For this review, take the finished solid that the model builds, in its own axes (mm). Round coordinates to 2 decimals unless told otherwise and drop trailing zeros. Write each loop counter-clockwise with the first axis right and the second up, starting at its lowest first coordinate (ties: lowest second). Pieces come first, ordered by that corner, then holes. Notation, with made-up numbers: (-33, -11.5) -> (0, -11.5) arc R19 ccw to (0, 25.5) -> close; hole circle Ø5 at (40.5, -15.5). An arc over 180 degrees is marked (long way). Answer in a Markdown table with one row per item. Add a question column.
Autodesk Inventor part; units mm, degrees
ref_plane "YZ Plane" through (0, 0, 0) normal (1, 0, 0) x (0, 1, 0)
ref_plane "XZ Plane" through (0, 0, 0) normal (0, 1, 0) x (-1, 0, 0)
ref_plane "XY Plane" through (0, 0, 0) normal (0, 0, 1) x (1, 0, 0)
sketch "Sketch1" plane through (0, 0, 0) normal (0, 0, 1) x (1, 0, 0)
  circle A0 centre (65.1069, 65.1069) radius 38.1 construction
  circle A1 centre (-56.1266, -56.1266) radius 25.4 construction
  circle A2 centre (0, 0) radius 53.975 construction
  line L0 (-38.1661, -38.1661) -> (38.1661, 38.1661) construction
  line L1 (65.1069, 65.1069) -> (-56.1266, -56.1266) construction
  line L2 (-4.3707, 6.2419) -> (-4.3707, 53.7978) construction
  line L3 (-213.7812, -81.5266) -> (651.6109, -81.5266) construction
  circle A3 centre (160.9392, -24.3766) radius 57.15 construction
  circle A4 centre (65.1069, 65.1069) radius 14.2875
  circle A5 centre (-56.1266, -56.1266) radius 14.2875
  circle A6 centre (-4.3707, 6.2419) radius 57.15 construction
  circle A7 centre (-56.1266, -56.1266) radius 20.6375 construction
  circle A8 centre (65.1069, 65.1069) radius 23.8125 construction
  circle A9 centre (-73.6972, 80.6773) radius 14.2875
  line L4 (-73.6972, 80.6773) -> (65.1069, 65.1069) construction
  circle A10 centre (65.1069, 65.1069) radius 14.3256 construction
  circle A11 centre (-56.1266, -56.1266) radius 14.3256 construction
  circle A12 centre (-109.5316, 9.8231) radius 14.2875
  line L5 (-56.1266, -56.1266) -> (-109.5316, 9.8231) construction
  circle A13 centre (-109.5316, 9.8231) radius 39.7002 construction
  circle A14 centre (-73.6972, 80.6773) radius 39.7002 construction
  line L6 (17.4877, 59.0466) -> (55.9992, 43.1049)
  line L7 (-39.0193, -44.5834) -> (-51.7448, -25.7239)
  arc A15 (17.4877, 59.0466) -> (-51.7448, -25.7239) centre (-4.3707, 6.2419) ccw
  line L8 (-178.6215, 120.6011) -> (-153.6074, 116.1905) construction
  line L9 (-153.6074, 116.1905) -> (-180.0714, -33.8943) construction
  line L10 (-180.0714, -33.8943) -> (-205.0855, -29.4836) construction
  line L11 (-205.0855, -29.4836) -> (-178.6215, 120.6011) construction
  line L12 (-209.5607, -54.8639) -> (48.3188, -100.335) construction
  line L13 (-174.1463, 145.9814) -> (151.5491, 88.5525) construction
  line L14 (-174.1463, 145.9814) -> (-209.5607, -54.8639) construction
  circle A16 centre (-138.9335, 44.7481) radius 25.4 construction
  circle A17 centre (-138.9335, 44.7481) radius 5.9531 construction
  line L15 (-84.5475, -21.0298) -> (-72.1113, -36.3871) construction
  circle A18 centre (17.7787, 70.4159) radius 9.525 construction
  line L16 (-166.1144, 118.3958) -> (-192.5784, -31.6889) construction
  line L17 (-170.5251, 93.3817) -> (-188.1678, -6.6748) construction
  circle A19 centre (-138.9335, 44.7481) radius 17.4625 construction
  circle A20 centre (-138.9335, 44.7481) radius 9.525 construction
  circle A21 centre (-73.6972, 80.6773) radius 46.0502 construction
  line L18 (-178.6215, 120.6011) -> (-76.4165, 126.6471)
  line L19 (-61.3431, 125.0394) -> (71.4951, 88.0465)
  line L20 (-62.4968, -75.7563) -> (-205.0855, -29.4836)
  line L21 (-178.6215, 120.6011) -> (-205.0855, -29.4836)
  arc A22 (-61.3431, 125.0394) -> (-76.4165, 126.6471) centre (-73.6972, 80.6773) ccw
  arc A23 (55.9992, 43.1049) -> (71.4951, 88.0465) centre (65.1069, 65.1069) ccw
  arc A24 (-62.4968, -75.7563) -> (-39.0193, -44.5834) centre (-56.1266, -56.1266) ccw
  line L22 (-138.9335, 44.7481) -> (-128.9174, 59.0525) construction
  line L23 (-121.633, 69.4558) -> (-156.234, 20.0404) construction
  circle A25 centre (-156.234, 20.0404) radius 4.7625 construction
  line L24 (-4.3707, 6.2419) -> (0, 0) construction
  circle A26 centre (-73.6972, 80.6773) radius 40.4812 construction
  circle A27 centre (-109.5316, 9.8231) radius 40.4812 construction
  circle A28 centre (-138.9335, 44.7481) radius 26.1938
  point P0 (-191.8535, 45.5588)
  point P1 (-78.3294, -28.7084)
  point P2 (-179.3464, 43.3534)
  point P3 (-179.3464, 43.3534)
  point P4 (-146.3135, 60.5745)
  point P5 (-156.3295, 46.2701)
  point P6 (-148.9496, 30.4437)
  point P7 (-131.5535, 28.9217)
  point P8 (-121.5374, 43.2261)
  point P9 (-63.3695, 121.1474)
  dimension "d7" = 50.8
  dimension "d18" = 79.4004
  dimension "d34" = 34.925
  dimension "d3" = 45
  dimension "d4" = 0
  dimension "d8" = 107.95
  dimension "d9" = 28.575
  dimension "d10" = 76.2
  dimension "d11" = 114.3
  dimension "d12" = 114.3
  dimension "d13" = 6.35
  dimension "d14" = 9.525
  dimension "d15" = 139.6746
  dimension "d16" = 28.6512
  dimension "d17" = 84.8614
  dimension "d19" = 79.4004
  dimension "d22" = 25.4
  dimension "d23" = 152.4
  dimension "d26" = 203.9436
  dimension "d27" = 50.8
  dimension "d28" = 11.9062
  dimension "d29" = 51
  dimension "d30" = 171.45
  dimension "d31" = 10
  dimension "d32" = 19.05
  dimension "d33" = 101.6
  dimension "d35" = 19.05
  dimension "d36" = 6.35
  dimension "d37" = 34.925
  dimension "d40" = 360
  dimension "d43" = 25
  dimension "d44" = 9.525
  dimension "d54" = 7.62
  dimension "d55" = 80
  dimension "d57" = 80.9625
  dimension "d59" = 0.7937
extrude "Extrusion1" add sketch "Sketch1" along normal blind 6.35
hole "Hole1" at (-78.3294, -28.7084, 0) at (17.7787, 70.4159, 0) at (-170.5251, 93.3817, 0) at (-179.3464, 43.3534, 0) at (-188.1678, -6.6748, 0) at (-128.9174, 59.0525, 0) at (-146.3135, 60.5745, 0) at (-156.3295, 46.2701, 0) at (-148.9496, 30.4437, 0) at (-131.5535, 28.9217, 0) at (-121.5374, 43.2261, 0) at (-121.633, 69.4558, 0) at (-156.234, 20.0404, 0) direction (0, 0, 1) diameter 5.1054 end through all
properties part number "GP7-002" material "Polycarbonate, Smoke"
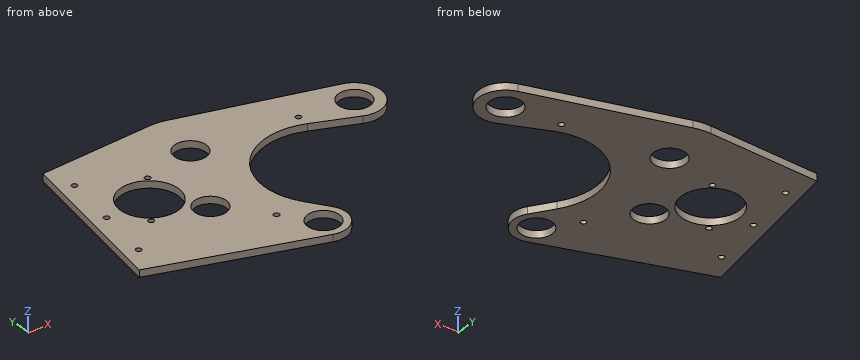
1. We need section B-B (y = 37). Write out the cut boundary in (x, z).
2. Clearance check with flat-ended pins moving along their axes: pin 1 Ø23 at (x, y) = (65.11, 65.11) entering from +Z; pin 2 Ø1.5 at (x, z) = (42.5, 0.5) entering from -Y; pin 3 Ø3 at (x, z) = (-63, 2) entering from +Y; pin 4 Ø2 at (x, z) = (-33.5, 3) entering from -Y. State where each tip first meets the part, or that it passes through.
3. We need section C-C (z = 2). Count the separate pieces of the cut face and the enclosed holes in it, plus the area to 3 significant figures.
4. We need section A-A (x = -144). Write out the cut boundary in (y, z).
5. We need section D-D (y = -21). Write out the cut boundary in (x, z).
6. For L1, parallel to Y at x = -67.5, z = 5.75; L2, parallel to X at y = 47, z = 6; L3, parallel to Y at x = -157, z = 3, list the stretches that pass through material, from the lowest coordinate up. Write a range as [from, to].
Response:
| question | item | result |
|---|---|---|
| 1 | outline | (-193.36, 0) -> (-163.96, 0) -> (-163.96, 6.35) -> (-193.36, 6.35) -> close; (-113.91, 0) -> (-52.54, 0) -> (-52.54, 6.35) -> (-113.91, 6.35) -> close |
| 2 | pin 1 | through |
| 2 | pin 2 | y = 48.38 |
| 2 | pin 3 | y = 125.8 |
| 2 | pin 4 | y = 54.8 |
| 3 | separate pieces | 1 |
| 3 | enclosed holes | 12 |
| 3 | area | 27,400 mm2 |
| 4 | outline | (-49.31, 0) -> (19.05, 0) -> (19.05, 6.35) -> (-49.31, 6.35) -> close; (70.45, 0) -> (122.65, 0) -> (122.65, 6.35) -> (70.45, 6.35) -> close |
| 5 | outline | (-203.59, 0) -> (-54.61, 0) -> (-54.61, 6.35) -> (-203.59, 6.35) -> close |
| 6 | L1 | [-74.13, -64.77], [-47.48, 67.8], [93.55, 126.31] |
| 6 | L2 | [-191.6, -165.03], [-112.84, -44.43], [46.59, 80.57] |
| 6 | L3 | [-45.09, 17.61], [22.48, 25.78], [63.71, 121.88] |
